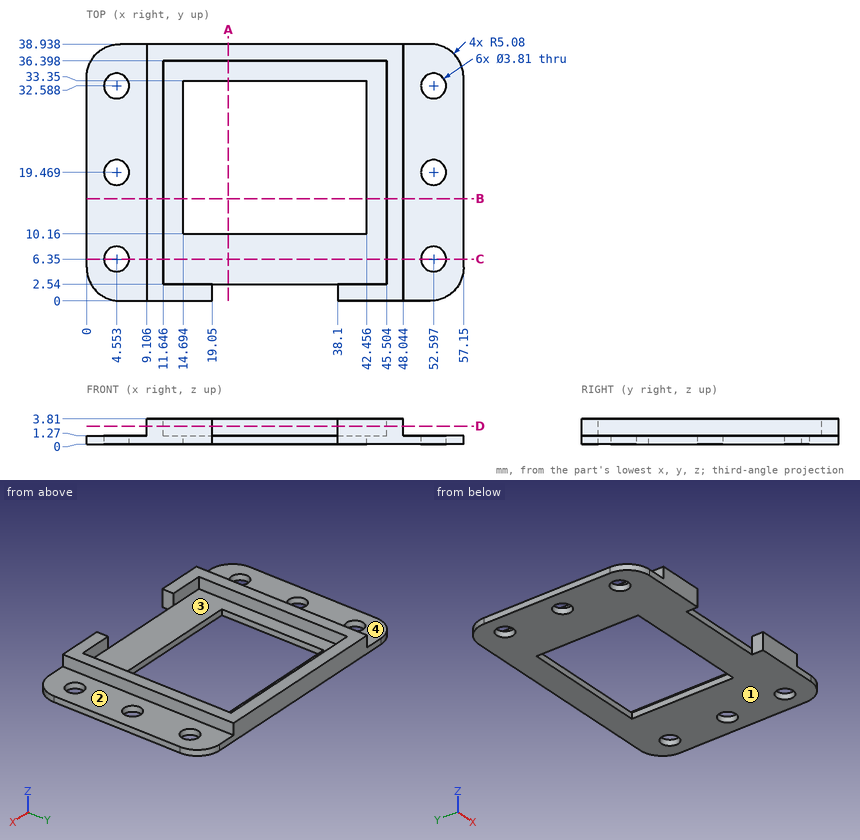
Could you check a few things on this drawing? It's one solid part, dimensions in mm from its lowest x, y, z. A direction names the side the tool comes from. Give positions to 0.01 mm unless a question says otherwise; leave off trailing zeros. Loops run counter-clockwise (first coordinate to the right, second up) from the corner with the lowest first, then second, coordinate; pieces in that order, holes last. Notation, with made-up numbers: M -8,55 L 17,55 A14 cw 17,63 Z; hole C -32.5,-18.5 d6. An arc over 180 degrees is marked long. Return JSON: item names as keys, results as strings.
Item 1: Imagine slicing it at A-A on x = 21.5. List the corners of the cut face in (y, z) for me.
A:
{"outline": "M 2.54,0 L 10.16,0 L 10.16,1.27 L 2.54,1.27 Z; M 33.35,0 L 38.94,0 L 38.94,3.81 L 36.4,3.81 L 36.4,1.27 L 33.35,1.27 Z"}
Item 2: On a 3-axis mill with a long thin cutter (end or side, diameter ignored), from which of +Z, -Z, +X, -X, +Y, -Y can I reach the whole of each face in a straight line? I mean the marked faces 1 and 2. Say none if no direction works.
A:
{"face 1": "-Z, +X, -X, +Y, -Y", "face 2": "+Z, +X, +Y, -Y"}
Item 3: I'm going to push flat-ended pins straight in: pin 1 Ø10 at (x, y) = (27, 24) entering from +Z; pin 2 Ø2.5 at (x, y) = (53.5, 26) entering from +Z; pin 3 Ø2 at (y, z) = (12.5, 3) entering from -X; pin 4 Ø1.4 at (x, z) = (24.5, 0.5) entering from -Y. Where does each tip first touch, or does it pass through?
A:
{"pin 1": "passes through", "pin 2": "stops at z = 1.27", "pin 3": "stops at x = 9.11", "pin 4": "stops at y = 2.54"}
Item 4: Thinking about a two-plate mould opening in Y: for the marked faces 3 and 4, which applies, released by +Y, released by -Y, zero draft, split by the parting line, or undercut?
A:
{"face 3": "undercut", "face 4": "zero draft"}
Item 5: Imagine slicing it at C-C on y = 6.35. List the corners of the cut face in (x, z) for me.
A:
{"outline": "M 0,0 L 2.65,0 L 2.65,1.27 L 0,1.27 Z; M 6.46,0 L 50.69,0 L 50.69,1.27 L 48.04,1.27 L 48.04,3.81 L 45.5,3.81 L 45.5,1.27 L 11.65,1.27 L 11.65,3.81 L 9.11,3.81 L 9.11,1.27 L 6.46,1.27 Z; M 54.5,0 L 57.15,0 L 57.15,1.27 L 54.5,1.27 Z"}
Item 6: Please list where these lines run through material, in increasing order: line 1 (X direction, y = 33, z = 2.45); line 2 (Y direction, x = 3.5, z = 0.65) (1 decimal); line 3 (X direction, y = 11, z = 1).
A:
{"line 1": "x = 9.11 to 11.65, 45.5 to 48.04", "line 2": "y = 0.3 to 4.8, 7.9 to 17.9, 21.1 to 31, 34.2 to 38.7", "line 3": "x = 0 to 14.69, 42.46 to 57.15"}
Item 7: Imagine slicing it at D-D on z = 2.7. List the corners of the cut face in (x, y) for me.
A:
{"outline": "M 9.11,0 L 19.05,0 L 19.05,2.54 L 11.65,2.54 L 11.65,36.4 L 45.5,36.4 L 45.5,2.54 L 38.1,2.54 L 38.1,0 L 48.04,0 L 48.04,38.94 L 9.11,38.94 Z"}
Item 8: Imagine slicing it at B-B on y = 15.5. List the corners of the cut face in (x, z) for me.
A:
{"outline": "M 0,0 L 14.69,0 L 14.69,1.27 L 11.65,1.27 L 11.65,3.81 L 9.11,3.81 L 9.11,1.27 L 0,1.27 Z; M 42.46,0 L 57.15,0 L 57.15,1.27 L 48.04,1.27 L 48.04,3.81 L 45.5,3.81 L 45.5,1.27 L 42.46,1.27 Z"}
